from build123d import *

# Parameters (mm, degrees)
BOSS_EXTRUDE1_DEPTH = 5
SKETCH2_R           = 17.5
SKETCH2_R_2         = 12.5
BOSS_EXTRUDE2_DEPTH = 70


with BuildPart() as part:
    # Sketch1 → Boss-Extrude1 (new body)
    with BuildSketch(Plane(origin=(0, 0, 0), x_dir=(1, 0, 0), z_dir=(0, 1, 0))):
        with BuildLine():
            Line((0, 0), (97.75, 0))
            Line((97.75, 0), (117.746979772, 19.996979772))
            Line((117.746979772, 19.996979772), (117.746979772, 49.996979772))
            Line((117.746979772, 49.996979772), (130.000479502, 49.996979772))
            Line((130.000479502, 49.996979772), (130.000479502, 119.996979772))
            Line((130.000479502, 119.996979772), (117.750479502, 119.996979772))
            Line((117.750479502, 119.996979772), (117.750479502, 139.999520498))
            Line((117.750479502, 139.999520498), (-39.999520498, 139.999520498))
            ThreePointArc((-39.999520498, 139.999520498), (-47.07058831, 137.07058831), (-49.999520498, 129.999520498))
            Line((-49.999520498, 129.999520498), (-49.999520498, 49.999520498))
            Line((-49.999520498, 49.999520498), (0, 0))
        make_face()
    extrude(amount=-BOSS_EXTRUDE1_DEPTH)

    # Sketch2 → Boss-Extrude2 (add)
    with BuildSketch(Plane(origin=(0, 0, -119.996979772), x_dir=(-1, 0, 0), z_dir=(0, 0, -1))):
        with Locations((-129.987472978, 12.499995167)):
            Circle(SKETCH2_R)
        with Locations((-129.987472978, 12.499995167)):
            Circle(SKETCH2_R_2, mode=Mode.SUBTRACT)
    extrude(amount=-BOSS_EXTRUDE2_DEPTH)


solid = part.part
Work out the finished part from the listing and answer in its coordinate system (mm). A direction names the side the tool comes from. Give positions to 0.01 mm unless a question says otherwise; leave off trailing zeros. Loops run counter-clockwise (first coordinate to the right, second up) from the corner with the lowest first, then second, coordinate; pieces in that order, holes last. Notation, with made-up numbers: (22.5, 63) - (69.5, 63) arc R21 cw to (69.5, 97) - close; hole circle Ø10 at (66, 88.5). An arc over 180 degrees is marked (long way). Answer in a Markdown table with one row per item. Add a question column.
Q1. The part is cut by section A-A (y = 20). Determine the outline of the cut face in (x, z).
Q2. A tool of negligible diameter and unlimited length cuts with its end or side. For faces 1 (the flat face through (117.75, -2, -130)), 2 (the flat face through (122, 1, -49.997)), 3 (the flat face through (122, 1, -119.997)), from which of +Z, -Z, +X, -X, +Y, -Y can it reach the whole face along a straight path? Write none if from no direction.
Q3. Consider line 1 along Y through (x, z) = (68, -39); line 2 along X through (y, z) = (14.5, -100.5); line 3 along X through (y, z) = (24, -60). Determine where each line is inside the solid, lowest interval first.
Q4. The part is cut by section C-C (x = 108.5). Determine the outline of the cut face in (y, z).
Q5. Each of these flat-tipped pins is pushed along its axis until it touches: P1, Ø5, axis at x = -5, z = -29.5, coming from the +Y side; P2, Ø15, axis at x = 129.99, y = 12.5, coming from the +Z side; P3, Ø2.5, axis at y = -2, z = -130, coming from the +X side; P4, Ø5.5, axis at y = -2.5, z = -31, coming from the +X side. Where does it stop, or does it pass through?
Q6. The part is cut by section D-D (z = -44). Determine the outline of the cut face in (x, y).
Solution:
| question | item | result |
|---|---|---|
| 1 | outline | (114.18, -120) - (119.99, -120) - (119.99, -50) - (114.18, -50) - close; (139.99, -120) - (145.8, -120) - (145.8, -50) - (139.99, -50) - close |
| 2 | face 1 | -Z, +X, +Y, -Y |
| 2 | face 2 | +Z, +X, +Y |
| 2 | face 3 | -Z, +X, +Y |
| 3 | line 1 | y = -5 to 0 |
| 3 | line 2 | x = 112.6 to 117.65, 142.33 to 147.37 |
| 3 | line 3 | x = 116.8 to 125.09, 134.89 to 143.18 |
| 4 | outline | (-5, -140) - (0, -140) - (0, -10.75) - (-5, -10.75) - close |
| 5 | P1 | stops at y = 0 |
| 5 | P2 | passes through |
| 5 | P3 | stops at x = 117.75 |
| 5 | P4 | stops at x = 117.75 |
| 6 | outline | (-44, -5) - (117.75, -5) - (117.75, 0) - (-44, 0) - close |
